Can you work these out from the drawing? Everything is in mm from the part's minimum corner. A direction names the side the tool comes from. Coordinates: 2 decimals unless noted, no trailing zeros. Loops run counter-clockwise (first coordinate to the right, second up) from the corner with the lowest first, then second, coordinate; pieces in that order, holes last. Notation, with made-up numbers: (75, 43) -> (96, 43) arc R26 cw to (96, 70) -> close; hole circle Ø8 at (89, -1). An arc over 180 degrees is marked (long way). Put each result on its own line as item: value. Start each with the question number.
Item 1: Please list where these lines run through material, in increasing order: L1, parallel to X at y = 6, z = 2.3; L2, parallel to X at y = 10.25, z = 0.95. Write a range as from..to.
Item 2: If we section it at B-B on z = 2.75: Please give me the cut outline in (x, y) (1 decimal).
Item 3: If we section it at A-A on x = 1: Please give me the cut outline in (y, z).
Item 4: If we section it at C-C on y = 12.5: Please give me the cut outline in (x, z).
Item 5: We'd pull the mould along Y, two halves only. Please class the marked faces 1, 2, 3 and 4: pulls with the +Y half, pulls with the -Y half, needs draft (parallel to the pull), parting line crosses it, or undercut.
Item 6: For the marked faces 5, 6 and 7, which set-ups out of +Z, -Z, +X, -X, +Y, -Y let a thin tool reach every point of the face, with its end or its side?
Item 7: If we section it at D-D on y = 1.5: Please give me the cut outline in (x, z).
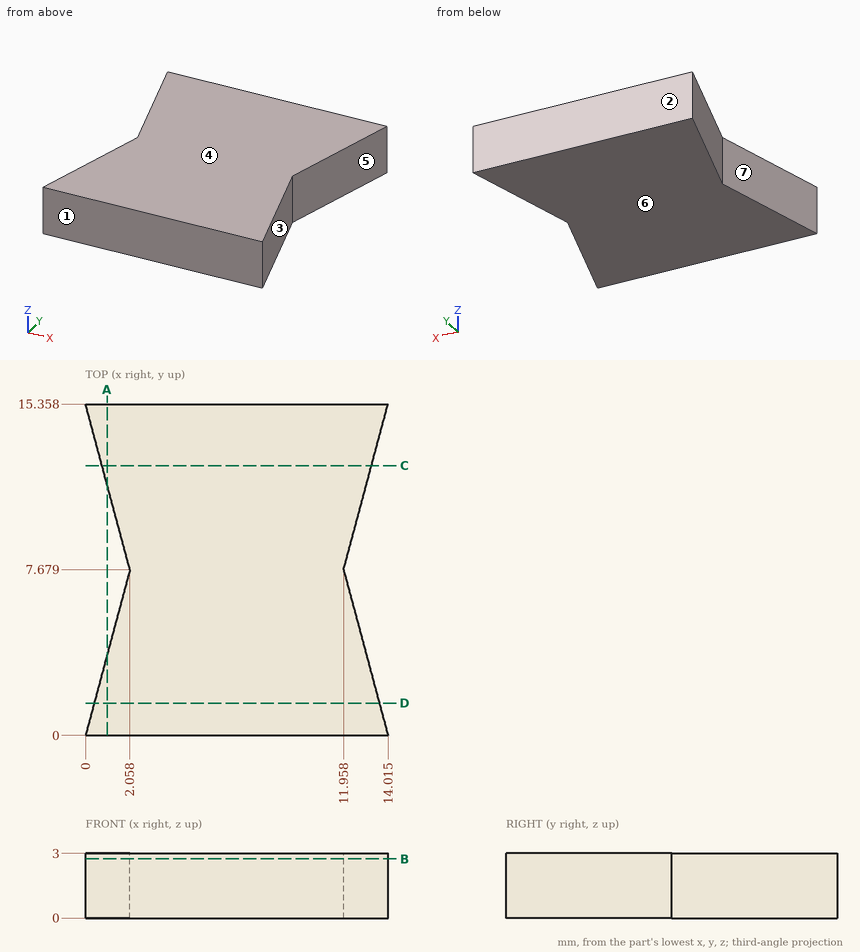
Solutions:
1. L1: 1.61..12.41
1. L2: 1.37..12.65
2. outline: (0, 0) -> (14, 0) -> (12, 7.7) -> (14, 15.4) -> (0, 15.4) -> (2.1, 7.7) -> close
3. outline: (0, 0) -> (3.73, 0) -> (3.73, 3) -> (0, 3) -> close; (11.63, 0) -> (15.36, 0) -> (15.36, 3) -> (11.63, 3) -> close
4. outline: (0.77, 0) -> (13.25, 0) -> (13.25, 3) -> (0.77, 3) -> close
5. face 1: pulls with the -Y half
5. face 2: pulls with the +Y half
5. face 3: undercut
5. face 4: needs draft
6. face 5: +Z, -Z, +X
6. face 6: -Z, +X, -X, +Y, -Y
6. face 7: +Z, -Z, -X
7. outline: (0.4, 0) -> (13.61, 0) -> (13.61, 3) -> (0.4, 3) -> close
